For this review, take the finished solid that the model builds, in its own axes (mm). Give positions to 0.01 mm unless a question says otherwise; leave off trailing zeros. Order: outer loops, then holes, each group sorted by start corner. A loop starts at its lowest first (then second) coordinate and runs counter-clockwise, first axis right, second up. Notation, with made-up numbers: (36, 81.25) -> (92, 81.25) arc R23 ccw to (92, 120.25) -> close; hole circle Ø7 at (4, -13.75). An arc over 180 degrees is marked (long way). One line per item, written item: value. Start each with the question number.
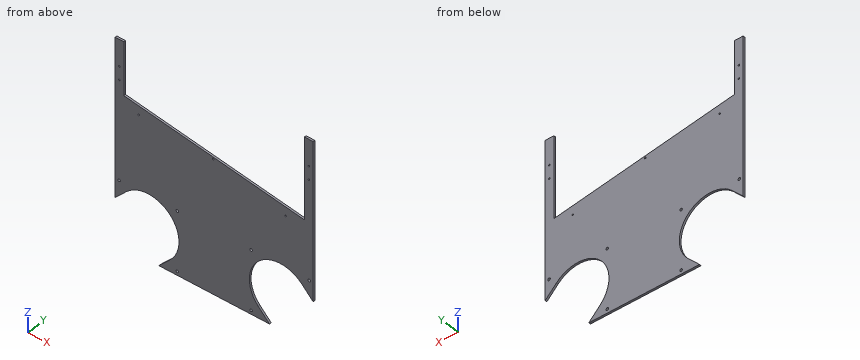
from build123d import *

# Parameters (mm, degrees)
BASE_FLANGE1_DEPTH    = 3
M3_TAPPED_HOLE1_D     = 2.5
M3_TAPPED_HOLE1_DEPTH = 7.5
M3_TAPPED_HOLE1_TIP   = 0.751075774
M3_TAPPED_HOLE2_D     = 2.5
M3_TAPPED_HOLE2_DEPTH = 7.5
M3_TAPPED_HOLE2_TIP   = 0.751075774
SKETCH11_R            = 47.5
SKETCH11_R_2          = 1.984375
CUT_EXTRUDE1_DEPTH    = 365.73826232


# Sheet-metal steps are written as plain solids
with BuildPart() as part:
    # Sketch1 → Base-Flange1 (new body)
    with BuildSketch(Plane(origin=(0, 0, 0), x_dir=(1, 0, 0), z_dir=(0, 1, 0))):
        Polygon((0, 0), (0, 200), (305, 200), (305, 35.309832976), (305, -105), (291.57115, -105), (291.57115, 18.045832093), (13.42885, -25), (13.42885, -105), (0, -105), align=None)
    extrude(amount=-BASE_FLANGE1_DEPTH)

    # M3 Tapped Hole1
    with Locations(Plane(origin=(0, 0, 0), x_dir=(1, 0, 0), z_dir=(0, 1, 0))):
        with Locations((6.5, -45), (6.5, -65), (298.5, -45), (298.5, -65)):
            Hole(M3_TAPPED_HOLE1_D / 2, depth=M3_TAPPED_HOLE1_DEPTH)
            with Locations((0, 0, -(M3_TAPPED_HOLE1_DEPTH + M3_TAPPED_HOLE1_TIP / 2))):  # 118° drill point
                Cone(0, M3_TAPPED_HOLE1_D / 2, M3_TAPPED_HOLE1_TIP, mode=Mode.SUBTRACT)

    # M3 Tapped Hole2
    with Locations(Plane(origin=(0, 0, 0), x_dir=(1, 0, 0), z_dir=(0, 1, 0))):
        with Locations((36.116318069, -8.031256885), (150.87789947, -0.629943868), (262.508000343, 27.005551046)):
            Hole(M3_TAPPED_HOLE2_D / 2, depth=M3_TAPPED_HOLE2_DEPTH)
            with Locations((0, 0, -(M3_TAPPED_HOLE2_DEPTH + M3_TAPPED_HOLE2_TIP / 2))):  # 118° drill point
                Cone(0, M3_TAPPED_HOLE2_D / 2, M3_TAPPED_HOLE2_TIP, mode=Mode.SUBTRACT)

    # Sketch11 → Cut-Extrude1 (cut, through all)
    with BuildSketch(Plane(origin=(0, 0, 0), x_dir=(1, 0, 0), z_dir=(0, 1, 0))):
        with BuildLine():
            Line((0, 200), (0, 132.824855788))
            Line((0, 132.824855788), (17.212427894, 115.612427894))
            ThreePointArc((17.212427894, 115.612427894), (17.212427894, 182.787572107), (84.387572107, 182.787572107))
            Line((84.387572107, 182.787572107), (67.175144213, 200))
            Line((67.175144213, 200), (0, 200))
        make_face()
        with Locations((50.8, 149.2)):
            Circle(SKETCH11_R)
        with Locations((254.2, 149.2)):
            Circle(SKETCH11_R)
        with BuildLine():
            Line((305, 200), (237.824855787, 200))
            Line((237.824855787, 200), (220.612427894, 182.787572106))
            ThreePointArc((220.612427894, 182.787572106), (272.377463037, 193.084277794), (301.7, 149.2))
            ThreePointArc((301.7, 149.2), (298.084277794, 131.022536963), (287.787572106, 115.612427894))
            Line((287.787572106, 115.612427894), (305, 132.824855787))
            Line((305, 132.824855787), (305, 200))
        make_face()
        with Locations(Location((95.6437, 194.0437, 0), (0, 0, 270))):
            Circle(SKETCH11_R_2)
        with Locations(Location((5.9563, 104.3563, 0), (0, 0, 270))):
            Circle(SKETCH11_R_2)
        with Locations(Location((95.6437, 104.3563, 0), (0, 0, 270))):
            Circle(SKETCH11_R_2)
        with Locations(Location((209.3563, 194.0437, 0), (0, 0, 270))):
            Circle(SKETCH11_R_2)
        with Locations(Location((209.3563, 104.3563, 0), (0, 0, 270))):
            Circle(SKETCH11_R_2)
        with Locations(Location((299.0437, 104.3563, 0), (0, 0, 270))):
            Circle(SKETCH11_R_2)
    extrude(amount=-CUT_EXTRUDE1_DEPTH, mode=Mode.SUBTRACT)


solid = part.part
Q1. For line 1 along X through (y, z) = (-2.5, 65); line 2 along X through (y, z) = (-1.4, 53.5); line 3 along Z through (x, y) = (6.5, -1.65), list the stretches that pass through material, from the lowest coordinate up.
Q2. Take a section at A-A (y = -1.75). State how many separate pieces and enclosed holes the cut face has, and give its area (3 significant figures).
Q3. Take a section at B-B (z = -149.2). State the section outline as (x, y) points, and give its area (3 significant figures).
Q4. For pin 1 Ø1.5 at (y, z) = (-2.5, -157) entering from -X, flat-tipped, find the tip position at first contact; note if it passes through.
Q5. Take a section at C-C (x = 202). State the section outline as (y, z) points, and give its area (3 significant figures).
Answers below:
1. line 1: x = 0 to 5.25, 7.75 to 13.43, 291.57 to 297.25, 299.75 to 305
1. line 2: x = 0 to 13.43, 291.57 to 305
1. line 3: z = -126.32 to -106.26, -102.45 to 43.75, 46.25 to 63.75, 66.25 to 105
2. separate pieces: 1
2. enclosed holes: 13
2. area: 48,500 mm²
3. outline: (98.3, -3) -> (206.7, -3) -> (206.7, 0) -> (98.3, 0) -> close
3. area: 325 mm²
4. pin 1: stops at x = 97.52
5. outline: (-3, -200) -> (0, -200) -> (0, -4.18) -> (-3, -4.18) -> close
5. area: 587 mm²
